```python
from build123d import *

# Parameters (mm, degrees)
SKETCH1_R           = 27.5
SKETCH1_R_2         = 2.5
BOSS_EXTRUDE1_DEPTH = 3.6
SKETCH2_R           = 20
SKETCH2_R_2         = 2.5
BOSS_EXTRUDE2_DEPTH = 15
SKETCH3_R           = 17.5
CUT_EXTRUDE1_DEPTH  = 5


with BuildPart() as part:
    # Sketch1 → Boss-Extrude1 (new body)
    with BuildSketch(Plane(origin=(0, 0, 0), x_dir=(1, 0, 0), z_dir=(0, 1, 0))):
        Circle(SKETCH1_R)
        with Locations((-9.959292144, 5.75)):
            Circle(SKETCH1_R_2, mode=Mode.SUBTRACT)
        with Locations((9.959292144, 5.75)):
            Circle(SKETCH1_R_2, mode=Mode.SUBTRACT)
        with Locations((0, -11.5)):
            Circle(SKETCH1_R_2, mode=Mode.SUBTRACT)
    extrude(amount=BOSS_EXTRUDE1_DEPTH)

    # Sketch2 → Boss-Extrude2 (add)
    with BuildSketch(Plane.XZ):
        Circle(SKETCH2_R)
        with Locations((0, 11.5)):
            Circle(SKETCH2_R_2, mode=Mode.SUBTRACT)
        with Locations((9.959292144, -5.75)):
            Circle(SKETCH2_R_2, mode=Mode.SUBTRACT)
        with Locations((-9.959292144, -5.75)):
            Circle(SKETCH2_R_2, mode=Mode.SUBTRACT)
    extrude(amount=BOSS_EXTRUDE2_DEPTH)

    # Sketch3 → Cut-Extrude1 (cut)
    with BuildSketch(Plane.XZ.offset(15)):
        Circle(SKETCH3_R)
    extrude(amount=-CUT_EXTRUDE1_DEPTH, mode=Mode.SUBTRACT)


solid = part.part
```
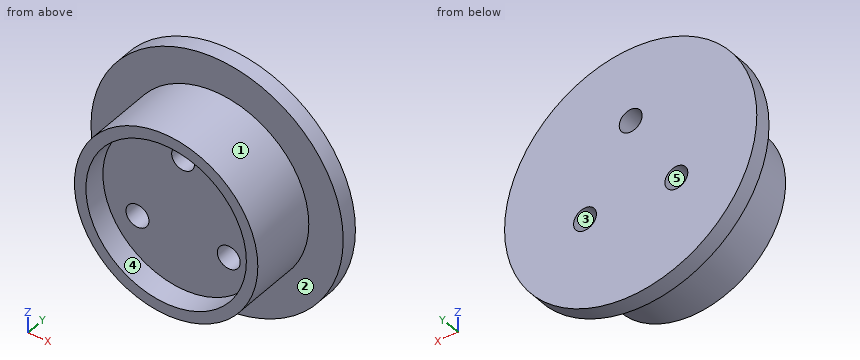
Design review of the part built by this model. Coordinates are the model's own, in mm. Face numbers are marked on the shaded views. A direction names the side the tool comes from. Give positions to 0.01 mm unless a question says otherwise; leave off trailing zeros. Write each loop counter-clockwise with the first axis right and the second up, starting at its lowest first coordinate (ties: lowest second). Pieces come first, ordered by that corner, then holes. Notation, with made-up numbers: (49.5, 40) - (96.5, 40) arc R14 cw to (96.5, 53) - close; hole circle Ø9 at (6, -16.5). An arc over 180 degrees is marked (long way). Return JSON: item names as keys, results as strings. Group by question number.
(1) Machinability: for the marked faces 4 and 5, which of the approach directions +Z, -Z, +X, -X, +Y, -Y give a long, thin tool a straight path to every point of the face, cutting with its end or side? Answer none if there is none.
(2) We need section D-D, the plane z = 11.5. Give the boundary of the cut face in (x, y).
(3) Mouldability with a two-part tool opening along X and no side actions: class the marked faces 1, 2 and 3 as +X half, -X half, draft (parallel to the pull), parting line (faces both ways), or undercut.
(4) We need section A-A, the plane x = 0. Give the boundary of the cut face in (y, z).
(5) We need section B-B, the plane z = -7. Give the boundary of the cut face in (x, y) (3 decimals).
(6) We need section C-C, the plane y = -10.75. Give the boundary of the cut face in (x, z).
(7) Insertion check: pin 1 (6.5 mm diameter, centred on x = 0, z = 11.5, fed in from -Y); pin 2 (8 mm diameter, centred on x = 5.5, y = -11, fed in from +Z); pin 3 (1 mm diameter, centred on y = -6, z = -4.5, fed in from -X). Each pin has a flat end and moves straight along its axis. Give the tip position at first contact, or say it passes through.
(8) To check wall thickness, follow probe 1 along X at (y, z) = (-4.25, -5.75); probe 2 along Y at (x, z) = (-24, 7); probe 3 along Z at (x, y) = (0, -12.8). State the ranges of each line that lie inside material, in increasing order.
Reported:
{
 "1": {"face 4": "-Y", "face 5": "+Y, -Y"},
 "2": {"outline": "(-24.98, 0) - (-16.36, 0) - (-16.36, -15) - (-13.19, -15) - (-13.19, -10) - (-2.5, -10) - (-2.5, 3.6) - (-24.98, 3.6) - close; (2.5, -10) - (13.19, -10) - (13.19, -15) - (16.36, -15) - (16.36, 0) - (24.98, 0) - (24.98, 3.6) - (2.5, 3.6) - close"},
 "3": {"face 1": "parting line", "face 2": "draft", "face 3": "undercut"},
 "4": {"outline": "(-15, -20) - (0, -20) - (0, -27.5) - (3.6, -27.5) - (3.6, 9) - (-10, 9) - (-10, -17.5) - (-15, -17.5) - close; (-15, 17.5) - (-10, 17.5) - (-10, 14) - (3.6, 14) - (3.6, 27.5) - (0, 27.5) - (0, 20) - (-15, 20) - close"},
 "5": {"outline": "(-26.594, 0) - (-18.735, 0) - (-18.735, -15) - (-16.039, -15) - (-16.039, -10) - (-12.124, -10) - (-12.124, 3.6) - (-26.594, 3.6) - close; (-7.794, -10) - (7.794, -10) - (7.794, 3.6) - (-7.794, 3.6) - close; (12.124, -10) - (16.039, -10) - (16.039, -15) - (18.735, -15) - (18.735, 0) - (26.594, 0) - (26.594, 3.6) - (12.124, 3.6) - close"},
 "6": {"outline": "circle Ø40 at (0, 0); hole circle Ø35 at (0, 0)"},
 "7": {"pin 1": "stops at y = -10", "pin 2": "stops at z = 19.94", "pin 3": "stops at x = -19.6"},
 "8": {"probe 1": "x = -19.16 to -12.46, -7.46 to 7.46, 12.46 to 19.16", "probe 2": "y = 0 to 3.6", "probe 3": "z = -20 to -17.5, 17.5 to 20"}
}
